Answer from the drawing. Dimensions are ordinates in mm from the lowest x, y and z of the part. A direction names the side the tool comes from. Round coordinates to 2 decimals unless told otherwise and drop trailing zeros. Write each loop counter-clockwise with the first axis right and the second up, starting at its lowest first coordinate (ties: lowest second). Pieces come first, ordered by that corner, then holes. Notation, with made-up numbers: (62, 1) - (117, 1) arc R14 ccw to (117, 5) - close; hole circle Ø3 at (-12, 14.25). An arc over 180 degrees is marked (long way). One line per item, written item: value. Start each with the question number.
(1) A cutting plane is placed at B-B, the plane x = 17.5. Determine the outline of the cut face in (y, z).
(2) A cutting plane is placed at C-C, the plane y = 10.5. Determine the outline of the cut face in (x, z), plus the area to 3 significant figures.
(3) A cutting plane is placed at A-A, the plane x = 35.55. Determine the outline of the cut face in (y, z).
(4) For the marked faces 5, 6, 7 and 8, determine the directions among +Z, -Z, +X, -X, +Y, -Y from which every point of the face is accessible in a straight line to the end or side of a thin tool.
(5) A cutting plane is placed at D-D, the plane y = 38. Determine the outline of the cut face in (x, z), plus the area to 3 significant figures.
(6) Find the intervals of material crossed by L1, parallel to Y at x = 27.55, z = 5.25; L2, parallel to Y at x = 27.55, z = 11.3; L3, parallel to X at y = 12.7, z = 10.05, in increasing order.
(7) The mould has two halves that part along Y. Classify the marked faces 1, 2, 3 and 4: +Y half, -Y half, draft (parallel to the pull), parting line (faces both ways), or undercut.
(8) Flat-ended cylindrical pins translate along their axes: pin 1 Ø0.6 at (x, y) = (28, 12) entering from -Z; pin 2 Ø8 at (x, y) = (36.5, 60) entering from -Z; pin 3 Ø3 at (y, z) = (46.5, 6) entering from +X. Find the tip coordinate at first contact, or state that the pin passes through.
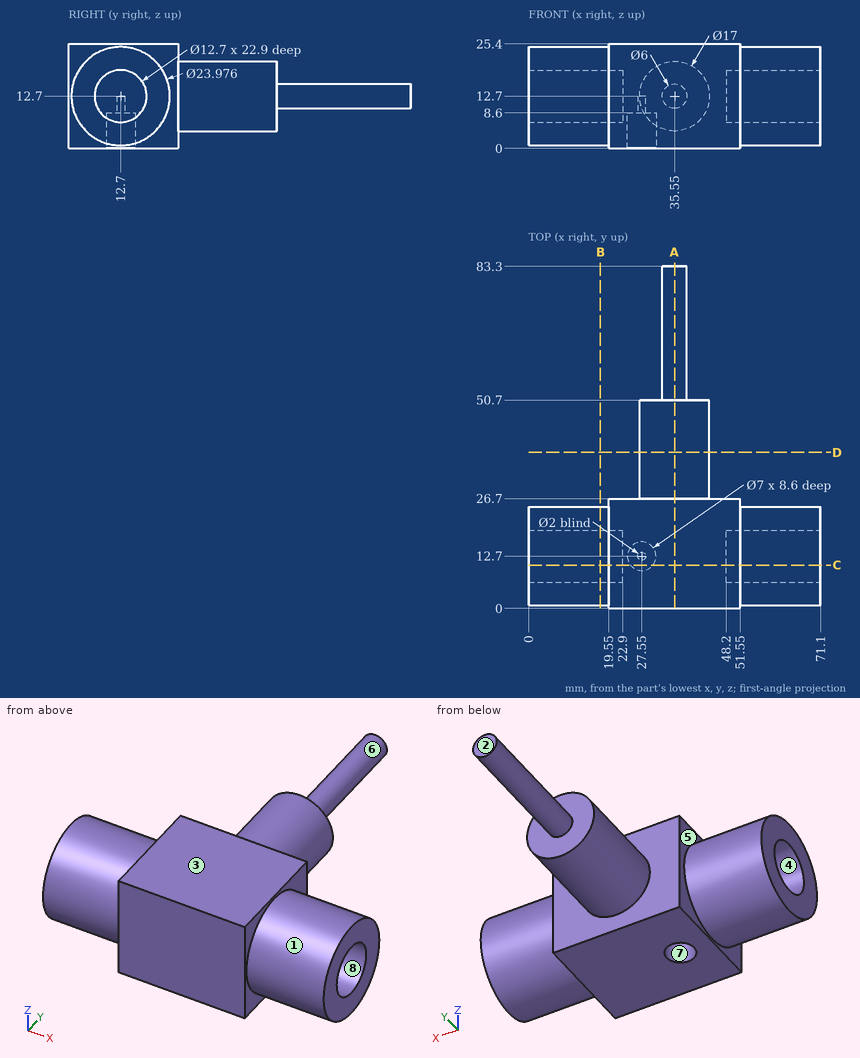
Here are the results:
1. outline: circle Ø23.98 at (12.7, 12.7); hole circle Ø12.7 at (12.7, 12.7)
2. outline: (0, 0.92) - (19.55, 0.92) - (19.55, 0) - (24.83, 0) - (24.83, 8.6) - (30.27, 8.6) - (30.27, 0) - (51.55, 0) - (51.55, 0.92) - (71.1, 0.92) - (71.1, 6.74) - (48.2, 6.74) - (48.2, 18.66) - (71.1, 18.66) - (71.1, 24.48) - (51.55, 24.48) - (51.55, 25.4) - (19.55, 25.4) - (19.55, 24.48) - (0, 24.48) - (0, 18.66) - (22.9, 18.66) - (22.9, 6.74) - (0, 6.74) - close
2. area: 1,140 mm²
3. outline: (0, 0) - (26.7, 0) - (26.7, 4.2) - (50.7, 4.2) - (50.7, 9.7) - (83.3, 9.7) - (83.3, 15.7) - (50.7, 15.7) - (50.7, 21.2) - (26.7, 21.2) - (26.7, 25.4) - (0, 25.4) - close
4. face 5: -X
4. face 6: +Y
4. face 7: -Z
4. face 8: +X
5. outline: circle Ø17 at (35.55, 12.7)
5. area: 227 mm²
6. L1: 0 to 9.2, 16.2 to 26.7
6. L2: 0 to 11.7, 13.7 to 50.7
6. L3: 22.9 to 26.55, 28.55 to 48.2
7. face 1: parting line
7. face 2: +Y half
7. face 3: draft
7. face 4: undercut
8. pin 1: z = 8.6
8. pin 2: z = 9.7
8. pin 3: x = 42.27
